Can you work these out from the drawing? Everything is in mm from the part's minimum corner. Round coordinates to 2 decimals unless told otherwise and drop trailing zeros. Loops run counter-clockwise (first coordinate to the right, second up) from the corner with the lowest first, then second, coordinate; pieces in that order, holes last. Notation, with made-up numbers: (53, -23.5) -> (110, -23.5) arc R37 cw to (110, 12.5) -> close; hole circle Ø5 at (-22.75, 12). An arc over 180 degrees is marked (long way). One line per item, written item: value.
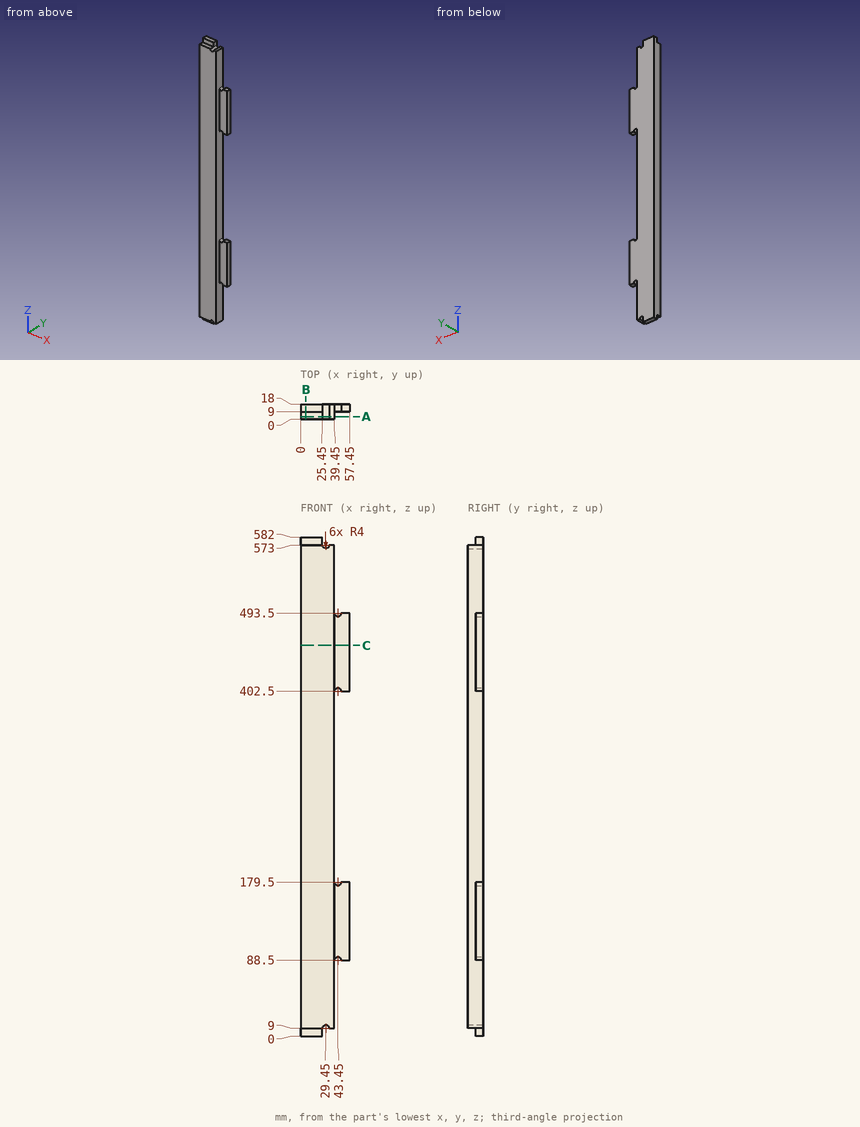
(1) If we section it at C-C, the plane z = 456: Please give me the cut outline in (x, y), then the cut area to 3 significant figures.
Recorded:
outline: (0, 0) -> (39.45, 0) -> (39.45, 9) -> (57.45, 9) -> (57.45, 18) -> (0, 18) -> close
area: 872 mm²
(2) If I drill on L1, parallel to Z at x = 55, y = 12.25; L2, parallel to X at y = 11.5, z = 76; L3, parallel to Z at x = 38, y = 7, over which ranges is the centre line in solid material (lowest first)?
Recorded:
L1: 88.5 to 179.5, 402.5 to 493.5
L2: 0 to 39.45
L3: 9 to 573
(3) If we section it at B-B, the plane x = 6: Please give me the cut outline in (y, z), then the cut area to 3 significant figures.
Recorded:
outline: (0, 9) -> (9, 9) -> (9, 0) -> (18, 0) -> (18, 582) -> (9, 582) -> (9, 573) -> (0, 573) -> close
area: 10,300 mm²
(4) If we section it at A-A, the plane y = 3.25: Please give me the cut outline in (x, z), then the cut area to 3 significant figures.
Recorded:
outline: (0, 9) -> (25.45, 9) arc R4 cw to (33.45, 9) -> (39.45, 9) -> (39.45, 573) -> (33.45, 573) arc R4 cw to (25.45, 573) -> (0, 573) -> close
area: 22,200 mm²
(5) I'm going to push flat-ended pins straight in: pin 1 Ø5 at (x, y) = (35.5, 6.5) entering from -Z; pin 2 Ø3 at (x, y) = (35.5, 10.5) entering from +Z; pin 3 Ø1 at (x, y) = (27, 9) entering from +Z. Where does each tip first touch, or does it pass through?
Recorded:
pin 1: z = 9
pin 2: z = 573
pin 3: z = 570.3
